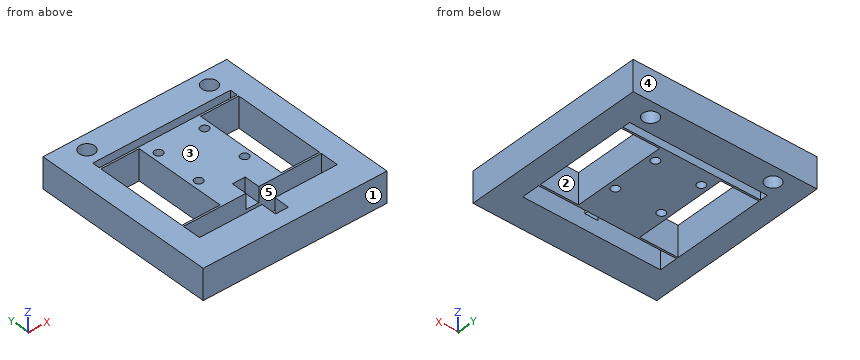
from build123d import *

# Parameters (mm, degrees)
SKETCH1_W                       = 76.2
SKETCH1_H                       = 76.2
BOSS_EXTRUDE1_DEPTH             = 6.35
SKETCH2_W                       = 57.15
SKETCH2_H                       = 3.175
SKETCH2_W_2                     = 15.875
SKETCH2_H_2                     = 38.481
SKETCH2_H_3                     = 7.62
CUT_EXTRUDE1_DEPTH              = 13.7
SKETCH3_W                       = 5.334
SKETCH3_H                       = 20.574
CUT_EXTRUDE2_DEPTH              = 6.35
F_1_4_0_25_DIAMETER_HOLE1_D     = 6.35
F_1_4_0_25_DIAMETER_HOLE1_DEPTH = 12.7
F_8_32_TAPPED_HOLE1_D           = 3.4544
F_8_32_TAPPED_HOLE1_DEPTH       = 12.7


with BuildPart() as part:
    # Sketch1 → Boss-Extrude1 (new body, symmetric)
    with BuildSketch(Plane.XY):
        Rectangle(SKETCH1_W, SKETCH1_H)
    extrude(amount=BOSS_EXTRUDE1_DEPTH, both=True)

    # Sketch2 → Cut-Extrude1 (cut, through all)
    with BuildSketch(Plane.XY.offset(6.35)):
        with Locations((0, 23.8125)):
            Rectangle(SKETCH2_W, SKETCH2_H)
        with Locations((20.6375, 2.2225)):
            Rectangle(SKETCH2_W_2, SKETCH2_H_2)
        with Locations((-20.6375, 2.2225)):
            Rectangle(SKETCH2_W_2, SKETCH2_H_2)
        with Locations((0, -21.59)):
            Rectangle(SKETCH2_W, SKETCH2_H_3)
    extrude(amount=-CUT_EXTRUDE1_DEPTH, mode=Mode.SUBTRACT)

    # Sketch3 → Cut-Extrude2 (cut)
    with BuildSketch(Plane.XY.offset(6.35)):
        with Locations((0, -21.59)):
            Rectangle(SKETCH3_W, SKETCH3_H)
    extrude(amount=-CUT_EXTRUDE2_DEPTH, mode=Mode.SUBTRACT)

    # 1/4 (0.25) Diameter Hole1
    with Locations(Plane.XY.offset(6.35)):
        with Locations((-25.4, 31.75), (25.4, 31.75)):
            Hole(F_1_4_0_25_DIAMETER_HOLE1_D / 2, depth=F_1_4_0_25_DIAMETER_HOLE1_DEPTH)

    # #8-32 Tapped Hole1
    with Locations(Plane.XY.offset(6.35)):
        with Locations((-9.525, 15.875), (9.525, 15.875), (9.525, -3.175), (-9.525, -3.175)):
            Hole(F_8_32_TAPPED_HOLE1_D / 2, depth=F_8_32_TAPPED_HOLE1_DEPTH)


solid = part.part
Could you check a few things on this model? Use its own coordinates, in mm. Face numbers are marked on the shaded views. A direction names the side the tool comes from. Give positions to 0.01 mm unless a question says otherwise; leave off trailing zeros. Order: outer loops, then holes, each group sorted by start corner. A loop starts at its lowest first (then second) coordinate and runs counter-clockwise, first axis right, second up. Notation, with made-up numbers: (24.25, 31) -> (36.25, 31) arc R14 cw to (36.25, 36) -> close; hole circle Ø8 at (39.5, -30). An arc over 180 degrees is marked (long way). Answer in a Markdown table with one row per item. Add a question column.
Item 1: Imagine slicing it at D-D (x = 21). List the corners of the cut face in (y, z) for me (3 decimals), and give its area (3 significant figures).
Item 2: For the marked faces 1 and 2, which set-ups out of +Z, -Z, +X, -X, +Y, -Y let a thin tool reach every point of the face, with its end or its side?
Item 3: Imagine slicing it at C-C (y = -16). List the corners of the cut face in (x, z) for me (3 decimals).
Item 4: We'd pull the mould along Y, two halves only. Please class the marked faces 3, 4 and 5: pulls with the +Y half, pulls with the -Y half, needs draft (parallel to the pull), parting line crosses it, or undercut.
Item 5: I'm going to push a flat-ended pin straight in: P1, Ø2.5, axis at x = -1, y = -13, coming from the +Z side. Where does the tip first touch, or does it pass through?
Item 6: Imagine slicing it at B-B (y = 24.5). List the corners of the cut face in (x, z) for me (3 decimals), and give its area (3 significant figures).
Item 7: Imagine slicing it at A-A (x = -4). List the corners of the cut face in (y, z) for me (3 decimals).
Item 8: Please list where these lines run through material, in increasing order: probe 1 along Y at (x, z) = (-1.5, -2.75) (3 decimals); probe 2 along Y at (x, z) = (-21.5, -1.75) (3 decimals); probe 3 along X at (y, z) = (-6.5, 4.5) (3 decimals).
Result:
| question | item | result |
|---|---|---|
| 1 | outline | (-38.1, -6.35) -> (-25.4, -6.35) -> (-25.4, 6.35) -> (-38.1, 6.35) -> close; (-17.78, -6.35) -> (-17.018, -6.35) -> (-17.018, 6.35) -> (-17.78, 6.35) -> close; (21.463, -6.35) -> (22.225, -6.35) -> (22.225, 6.35) -> (21.463, 6.35) -> close; (25.4, -6.35) -> (38.1, -6.35) -> (38.1, 6.35) -> (25.4, 6.35) -> close |
| 1 | area | 342 mm2 |
| 2 | face 1 | +Z, -Z, +X, -X, -Y |
| 2 | face 2 | +Z, -Z |
| 3 | outline | (-38.1, -6.35) -> (-28.575, -6.35) -> (-28.575, 6.35) -> (-38.1, 6.35) -> close; (-12.7, -6.35) -> (12.7, -6.35) -> (12.7, 6.35) -> (2.667, 6.35) -> (2.667, 0) -> (-2.667, 0) -> (-2.667, 6.35) -> (-12.7, 6.35) -> close; (28.575, -6.35) -> (38.1, -6.35) -> (38.1, 6.35) -> (28.575, 6.35) -> close |
| 4 | face 3 | needs draft |
| 4 | face 4 | pulls with the +Y half |
| 4 | face 5 | undercut |
| 5 | P1 | z = 0 |
| 6 | outline | (-38.1, -6.35) -> (-28.575, -6.35) -> (-28.575, 6.35) -> (-38.1, 6.35) -> close; (28.575, -6.35) -> (38.1, -6.35) -> (38.1, 6.35) -> (28.575, 6.35) -> close |
| 6 | area | 242 mm2 |
| 7 | outline | (-38.1, -6.35) -> (-25.4, -6.35) -> (-25.4, 6.35) -> (-38.1, 6.35) -> close; (-17.78, -6.35) -> (22.225, -6.35) -> (22.225, 6.35) -> (-17.78, 6.35) -> close; (25.4, -6.35) -> (38.1, -6.35) -> (38.1, 6.35) -> (25.4, 6.35) -> close |
| 8 | probe 1 | -38.1 to -25.4, -17.78 to 22.225, 25.4 to 38.1 |
| 8 | probe 2 | -38.1 to -25.4, -17.78 to -17.018, 21.463 to 22.225, 25.4 to 38.1 |
| 8 | probe 3 | -38.1 to -28.575, -12.7 to 12.7, 28.575 to 38.1 |
